Geometry: see drawing. Coordinates: mm, zero at the bounding-box minimum. Coordinates: 2 decimals unless noted, no trailing zeros. Write each loop counter-clockwise with the first axis right and the second up, starting at its lowest first coordinate (ties: lowest second). Pieces come first, ordered by that corner, then holes. Notation, with made-up numbers: (38.25, 61) - (74.25, 61) arc R23 cw to (74.25, 86) - close; hole circle Ø4 at (79, 68). An arc over 180 degrees is marked (long way). One line per question, with ' | ' between items. Start each with the question number.
1) Section query D-D on z = 45.5. Return loops of the section in (x, y).
2) Section query B-B on x = 29.5. Return loops of the section in (y, z).
3) Section query A-A on z = 29.5. Return loops of the section in (x, y), and give its area (4 significant figures).
4) Section query C-C on y = 3.75. Return loops of the section in (x, z), and give its area (3 significant figures).
5) Draft query along X for the marked faces 1, 2 and 3. Return one class per face: released by +X, released by -X, zero draft, split by the parting line, or undercut.
6) First-contact query: P1, Ø1, axis at y = 6, z = 18, coming from the -X side; P2, Ø2, axis at y = 4, z = 26, coming from the +X side; P3, Ø2, axis at y = 7, z = 3, coming from the -X side. Flat tips, straight axial feed; report the tip coordinate or a pass-through.
7) Line query: line 1 (Z direction, x = 29.5, y = 0.65); line 2 (Y direction, x = 44.5, z = 46); line 3 (X direction, y = 3, z = 29). Output: solid intervals per line, ascending.
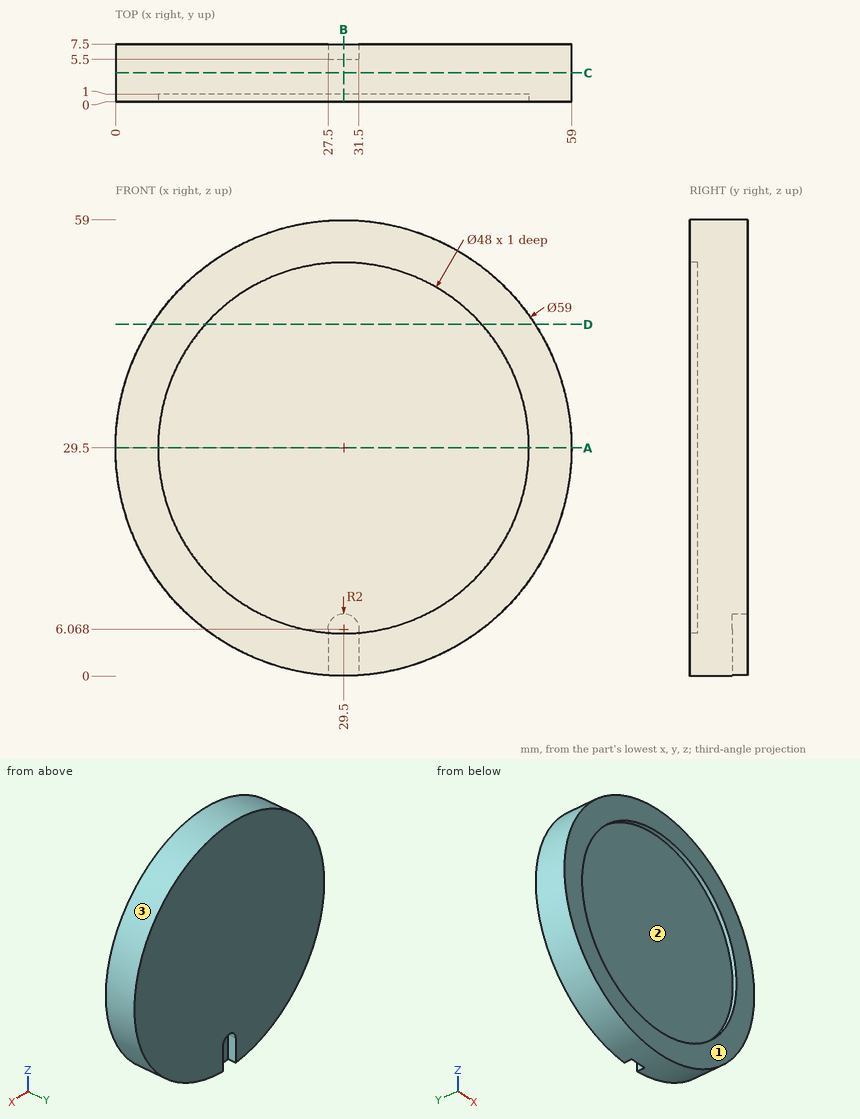
Answer key:
1) outline: (4.72, 0) - (11.61, 0) - (11.61, 1) - (47.39, 1) - (47.39, 0) - (54.28, 0) - (54.28, 7.5) - (4.72, 7.5) - close
2) outline: (0, 0) - (5.5, 0) - (5.5, 8.07) - (7.5, 8.07) - (7.5, 59) - (0, 59) - (0, 53.5) - (1, 53.5) - (1, 5.5) - (0, 5.5) - close
3) outline: (0, 0) - (5.5, 0) - (5.5, 1) - (53.5, 1) - (53.5, 0) - (59, 0) - (59, 7.5) - (0, 7.5) - close | area: 394.5 mm²
4) outline: circle Ø59 at (29.5, 29.5) | area: 2,730 mm²
5) face 1: zero draft | face 2: undercut | face 3: split by the parting line
6) P1: x = 2.13 | P2: x = 58.89 | P3: x = 14.67
7) line 1: 0 to 5.5, 53.5 to 59 | line 2: 1 to 7.5 | line 3: 0 to 59
